Input: part model. Units: mm. Frame: model coordinates. A direction names the side the tool comes from. Give positions to 0.01 mm unless a question says otherwise; leave off trailing zeros. Order: outer loops, then holes, each group sorted by start corner. A loop starts at its lowest first (then second) coordinate and runs counter-clockwise, first axis right, second up.
```python
from build123d import *

# Parameters (mm, degrees)
SKETCH1_R           = 1.5875
BOSS_EXTRUDE1_DEPTH = 9.398
SKETCH2_R           = 0.3429
BOSS_EXTRUDE2_DEPTH = 2.794
SKETCH3_W           = 1.27
SKETCH3_H           = 5.3848
BOSS_EXTRUDE3_DEPTH = 0.3048
SKETCH4_W           = 0.5842
SKETCH4_H           = 0.3048
BOSS_EXTRUDE4_DEPTH = 2.794
FILLET1_R           = 0.127
SKETCH5_R           = 1.237083483
CUT_EXTRUDE1_DEPTH  = 7.874


with BuildPart() as part:
    # Sketch1 → Boss-Extrude1 (new body)
    with BuildSketch(Plane(origin=(0, 0, 0), x_dir=(1, 0, 0), z_dir=(0, 1, 0))):
        with Locations(Location((0, 0, 0), (0, 0, 270))):
            Circle(SKETCH1_R)
    extrude(amount=BOSS_EXTRUDE1_DEPTH)

    # Sketch2 → Boss-Extrude2 (add)
    with BuildSketch(Plane(origin=(0, 0, 0), x_dir=(-1, 0, 0), z_dir=(0, -1, 0))):
        with Locations(Location((0, 0, 0), (0, 0, 270))):
            Circle(SKETCH2_R)
    extrude(amount=BOSS_EXTRUDE2_DEPTH)

    # Sketch3 → Boss-Extrude3 (add)
    with BuildSketch(Plane(origin=(0, 0, 0), x_dir=(-1, 0, 0), z_dir=(0, -1, 0))):
        Rectangle(SKETCH3_W, SKETCH3_H)
    extrude(amount=-BOSS_EXTRUDE3_DEPTH)

    # Sketch4 → Boss-Extrude4 (add)
    with BuildSketch(Plane(origin=(0, 0, 0), x_dir=(-1, 0, 0), z_dir=(0, -1, 0))):
        with Locations((0, 2.54)):
            Rectangle(SKETCH4_W, SKETCH4_H)
        with Locations((0, -2.54)):
            Rectangle(SKETCH4_W, SKETCH4_H)
    extrude(amount=BOSS_EXTRUDE4_DEPTH)

    # Fillet1
    fillet1_edges = [part.edges().sort_by_distance(p)[0] for p in [
        (0, 0.3048, 2.6924),
        (0, 0.3048, -2.6924),
    ]]
    fillet(fillet1_edges, radius=FILLET1_R)

    # Sketch5 → Cut-Extrude1 (cut)
    with BuildSketch(Plane(origin=(0, 9.398, 0), x_dir=(1, 0, 0), z_dir=(0, 1, 0))):
        with Locations(Location((0, 0, 0), (0, 0, 270))):
            Circle(SKETCH5_R)
    extrude(amount=-CUT_EXTRUDE1_DEPTH, mode=Mode.SUBTRACT)


solid = part.part
```
1) Pull-direction query (Z, two-part tool) for faces 1 (the face through (-0.966, 4.633, -1.26)), 2 (the face through (0, 0.305, 2)), 3 (the face through (0, 0, 1)), 4 (the face through (0, -1, 2.692)); classes: pulls with the +Z half, pulls with the -Z half, needs draft (parallel to the pull), parting line crosses it, or undercut.
2) Cut plane C-C (y = 8.25). Return the cut outline in (x, z) (1 decimal).
3) Cut plane D-D (z = -0.6). Return the cut outline in (x, y).
4) Cut plane B-B (z = 0). Return the cut outline in (x, y).
5) Line query: probe 1 along X at (y, z) = (8.5, 0); probe 2 along Y at (x, z) = (-0.5, -1.6); probe 3 along Y at (x, z) = (-0.6, 0.05). Output: solid intervals per line, ascending.
6) Reachability of faces 5 (the face through (0.37, 5.52, 1.18)), 6 (the face through (-1, 9.398, 1)) from +Z, -Z, +X, -X, +Y, -Y: full face, straight path, thin tool, end or side. Return the list, or none.
7) First-contact query: P1, Ø1.2, axis at x = 0, z = -2.5, coming from the +Y side; P2, Ø1.5, axis at y = -1.5, z = -0.5, coming from the -X side; P3, Ø1, axis at x = 0, z = 2, coming from the +Y side. Flat tips, straight axial feed; report the tip coordinate or a pass-through.
8) Cut plane A-A (x = 0). Return the cut outline in (y, z).
Geometry says:
1. face 1: parting line crosses it
1. face 2: needs draft
1. face 3: undercut
1. face 4: pulls with the +Z half
2. outline: circle Ø3.2 at (0, 0); hole circle Ø2.5 at (0, 0)
3. outline: (-1.47, 0) - (1.47, 0) - (1.47, 9.4) - (1.08, 9.4) - (1.08, 1.52) - (-1.08, 1.52) - (-1.08, 9.4) - (-1.47, 9.4) - close
4. outline: (-1.59, 0) - (-0.34, 0) - (-0.34, -2.79) - (0.34, -2.79) - (0.34, 0) - (1.59, 0) - (1.59, 9.4) - (1.24, 9.4) - (1.24, 1.52) - (-1.24, 1.52) - (-1.24, 9.4) - (-1.59, 9.4) - close
5. probe 1: x = -1.59 to -1.24, 1.24 to 1.59
5. probe 2: y = 0 to 0.3
5. probe 3: y = 0 to 1.52
6. face 5: +Y
6. face 6: +Z, -Z, +X, -X, +Y
7. P1: stops at y = 0.3
7. P2: stops at x = -0.34
7. P3: stops at y = 9.4
8. outline: (-2.79, -2.69) - (0.18, -2.69) arc R0.13 ccw to (0.3, -2.57) - (0.3, -1.59) - (9.4, -1.59) - (9.4, -1.24) - (1.52, -1.24) - (1.52, 1.24) - (9.4, 1.24) - (9.4, 1.59) - (0.3, 1.59) - (0.3, 2.57) arc R0.13 ccw to (0.18, 2.69) - (-2.79, 2.69) - (-2.79, 2.39) - (0, 2.39) - (0, 0.34) - (-2.79, 0.34) - (-2.79, -0.34) - (0, -0.34) - (0, -2.39) - (-2.79, -2.39) - close
